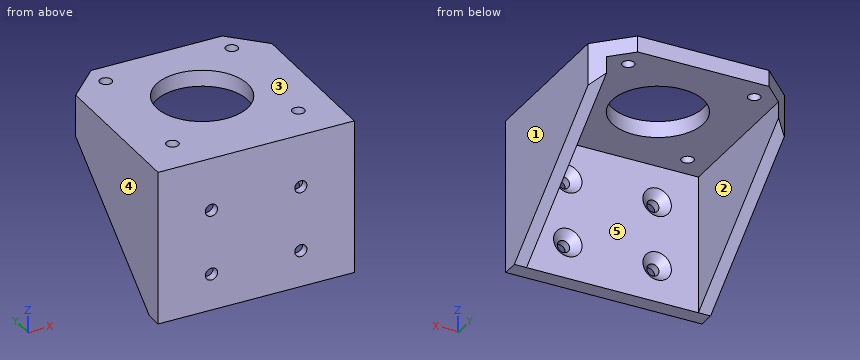
Autodesk Inventor part; units mm, degrees
ref_plane "YZ Plane" through (0, 0, 0) normal (1, 0, 0) x (0, 1, 0)
ref_plane "XZ Plane" through (0, 0, 0) normal (0, 1, 0) x (-1, 0, 0)
ref_plane "XY Plane" through (0, 0, 0) normal (0, 0, 1) x (1, 0, 0)
sketch "Szkic5" plane through (0, 0, 0) normal (1, 0, 0) x (0, 1, 0)
  line L0 (0, 0) -> (4, 0)
  line L1 (4, 0) -> (4, -38)
  line L2 (4, -38) -> (0, -38)
  line L3 (0, -38) -> (0, 0)
  line L4 (4, 0) -> (46.3, 0)
  line L5 (46.3, 0) -> (46.3, -4)
  line L6 (46.3, -4) -> (4, -4)
  line L7 (4, -4) -> (4, 0)
  dimension "d10" = 4
  dimension "d11" = 38
  dimension "d12" = 42.3
  dimension "d13" = 4
extrude "Wyciągnięcie proste2" add sketch "Szkic5" along normal blind 48.3
sketch "Szkic6" plane through (0, 4, -4) normal (0, 1, 0) x (1, 0, 0)
  line L0 (48.3, -4) -> (48.3, 34)
  line L1 (48.3, 34) -> (45.3, 34)
  line L2 (45.3, 34) -> (45.3, 0)
  line L3 (45.3, 0) -> (48.3, 0)
  line L4 (48.3, 0) -> (48.3, 34)
  line L5 (0, -4) -> (0, 34)
  line L6 (0, 34) -> (3, 34)
  line L7 (3, 34) -> (3, 0)
  line L8 (3, 0) -> (0, 0)
  line L9 (0, 0) -> (0, 34)
  dimension "d16" = 3
  dimension "d17" = 34
  dimension "d18" = 3
  dimension "d19" = 34
extrude "Wyciągnięcie proste3" add sketch "Szkic6" along normal blind 42.3
sketch "Szkic7" plane through (0, 0, 0) normal (-1, 0, 0) x (0, 0, 1)
  line L0 (-4, 46.3) -> (-38, 46.3)
  line L1 (-4, 46.3) -> (-38, 46.3)
  line L2 (-38, 4) -> (-38, 46.3)
  line L3 (-38, 46.3) -> (-38, 4)
  line L4 (-38, 4) -> (-4, 46.3)
  point P0 (0, 0)
extrude "Wyciągnięcie proste4" cut sketch "Szkic7" against normal through all
sketch "Szkic8" plane through (45.3, 4, -4) normal (0, 0, -1) x (-1, 0, 0)
  line L0 (45.3, 42.3) -> (-3, 42.3)
  line L1 (-3, 0) -> (-3, 42.3)
  line L2 (0, 42.3) -> (0, 0)
  circle A0 centre (21.15, 21.15) radius 11.25
  point P0 (45.3, -4)
  dimension "d24" = 21.15
  dimension "d26" = 21.15
  dimension "d27" = 22.5
extrude "Wyciągnięcie proste5" cut sketch "Szkic8" against normal blind 42.3
sketch "Szkic9" plane through (45.3, 4, -4) normal (0, 0, -1) x (-1, 0, 0)
  line L0 (45.3, 42.3) -> (-3, 42.3)
  line L1 (21.15, 42.3) -> (21.15, 0) construction
  line L2 (42.3, 0) -> (0, 0)
  line L3 (0, 42.3) -> (0, 0)
  line L4 (0, 21.15) -> (42.3, 21.15) construction
  line L5 (45.3, 42.3) -> (45.3, -4)
  point P0 (5.65, 36.65)
  point P1 (36.65, 36.65)
  point P2 (5.65, 5.65)
  point P3 (36.65, 5.65)
  dimension "d30" = 15.5
  dimension "d31" = 15.5
hole "Otwór1" at (39.65, 40.65, -4) at (8.65, 40.65, -4) at (39.65, 9.65, -4) at (8.65, 9.65, -4) direction (0, 0, 1) diameter 3 depth 8 tip angle 118
sketch "Szkic10" plane through (3, 4, -4) normal (0, 1, 0) x (1, 0, 0)
  line L0 (9.9, 0) -> (32.4, 0)
  line L1 (21.15, 0) -> (21.15, 34) construction
  line L2 (0, 34) -> (42.3, 34)
  line L3 (42.3, 0) -> (42.3, 34)
  line L4 (42.3, 17) -> (0, 17) construction
  line L5 (0, 34) -> (0, 0)
  point P0 (-3, -4)
  point P1 (32.15, 9)
  point P2 (10.15, 9)
  point P3 (32.15, 25)
  point P4 (10.15, 25)
  dimension "d39" = 11
  dimension "d40" = 8
hole "Otwór2" at (35.15, 4, -13) at (13.15, 4, -13) at (35.15, 4, -29) at (13.15, 4, -29) direction (0, -1, 0) diameter 3 depth 8 tip angle 118
chamfer "Faza1" distance 2 angle 45 4 edges at (35.15, 4, -14.5) (13.15, 4, -14.5) (35.15, 4, -30.5) (13.15, 4, -30.5)
chamfer "Faza2" distance 8 angle 45 2 edges at (48.3, 46.3, -2) (0, 46.3, -2)
properties part number "Ucwyt_NEMA17"
Model file for the job. Use its own axes, mm. Face numbers are marked on the shaded views. A direction names the side the tool comes from. Round coordinates to 2 decimals unless told otherwise and drop trailing zeros. Order: outer loops, then holes, each group sorted by start corner. A loop starts at its lowest first (then second) coordinate and runs counter-clockwise, first axis right, second up. Notation, with made-up numbers: M 23,-1 L 37,-1 A6 ccw 37,9 Z; hole C 44.25,44 d3. An arc over 180 degrees is marked long. Write each question's results on one line, items separated by ' | '. Start each with the question number.
(1) Saw through at B-B, the plane y = 25.15. Give the cut face in (x, z).
(2) Saw through at D-D, the plane y = 9.65. Give the cut face in (x, z).
(3) Drop flat-ended pins along their axis: pin 1 (2 mm diameter, centred on x = 15.5, y = 5.5, fed in from -Z); pin 2 (2 mm diameter, centred on x = 40.5, y = 11, fed in from +Z); pin 3 (12 mm diameter, centred on x = 35, z = -21.5, fed in from +Y); pin 4 (3.5 mm diameter, centred on x = 13.15, z = -29, fed in from +Y). Give the stop position or say it passes through.
(4) Saw through at C-C, the plane z = -13. Give the cut face in (x, y).
(5) Which spindle directions (+Z, -Z, +X, -X, +Y, -Y) get a long thin tool onto all of the face, cutting with end or side? Do the marked faces 1 and 2. Say none if no direction does.
(6) Two-plate mould, pull along X, no slides. Class the marked faces 3, 4 and 5: pulls with the +X half, pulls with the -X half, needs draft (parallel to the pull), parting line crosses it, or undercut.
(7) Saw through at A-A, the plane x = 8.65. Give the cut face in (y, z), then the cut area to 3 significant figures.
(8) Probe probe 1 along Y at (x, z) = (8.65, -1.8); probe 2 along X at (y, z) = (0.55, -29); probe 3 along Z at (x, y) = (35.15, 1.6). List the from-to ranges inside material, lowest first. Write a range as from..to.
Established:
1) outline: M 0,-21 L 3,-21 L 3,-4 L 12.9,-4 L 12.9,0 L 0,0 Z; M 35.4,-4 L 45.3,-4 L 45.3,-21 L 48.3,-21 L 48.3,0 L 35.4,0 Z
2) outline: M 0,-33.46 L 3,-33.46 L 3,-4 L 7.15,-4 L 7.15,0 L 0,0 Z; M 10.15,-4 L 38.15,-4 L 38.15,0 L 10.15,0 Z; M 41.15,-4 L 45.3,-4 L 45.3,-33.46 L 48.3,-33.46 L 48.3,0 L 41.15,0 Z
3) pin 1: stops at z = -4 | pin 2: stops at z = 0 | pin 3: stops at y = 4 | pin 4: stops at y = 2.25
4) outline: M 0,0 L 11.65,0 L 11.65,2 L 9.65,4 L 3,4 L 3,35.1 L 0,35.1 Z; M 14.65,0 L 33.65,0 L 33.65,2 L 31.65,4 L 16.65,4 L 14.65,2 Z; M 36.65,0 L 48.3,0 L 48.3,35.1 L 45.3,35.1 L 45.3,4 L 38.65,4 L 36.65,2 Z
5) face 1: +Z, -Z, +X, +Y, -Y | face 2: -Z, +Y
6) face 3: needs draft | face 4: pulls with the -X half | face 5: undercut
7) outline: M 0,-38 L 4,-38 L 4,-4 L 8.15,-4 L 8.15,0 L 0,0 Z; M 11.15,-4 L 39.15,-4 L 39.15,0 L 11.15,0 Z; M 42.15,-4 L 46.3,-4 L 46.3,0 L 42.15,0 Z | area: 297 mm^2
8) probe 1: y = 0..8.15, 11.15..39.15, 42.15..46.3 | probe 2: x = 0..11.65, 14.65..33.65, 36.65..48.3 | probe 3: z = -38..-30.5, -27.5..-14.5, -11.5..0
